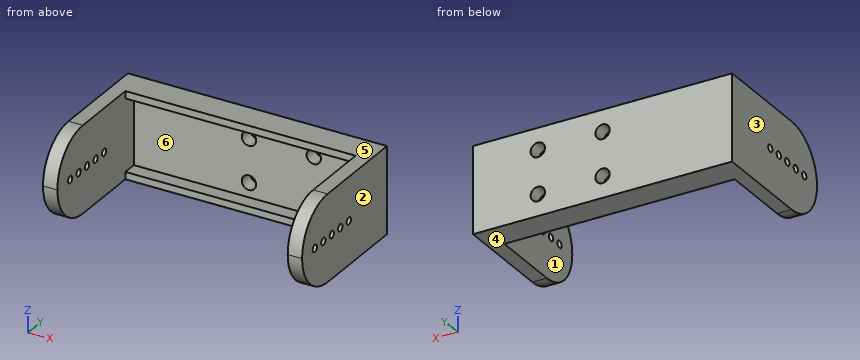
from build123d import *

# Parameters (mm, degrees)
SKETCH1_W           = 36
SKETCH1_H           = 20
BOSS_EXTRUDE1_DEPTH = 12
SKETCH3_W           = 32
SKETCH3_H           = 16
CUT_EXTRUDE1_DEPTH  = 12
SKETCH4_W           = 32
SKETCH4_H           = 12
CUT_EXTRUDE2_DEPTH  = 12
CUT_EXTRUDE3_DEPTH  = 40.242833741
SKETCH5_R           = 1
CUT_EXTRUDE4_DEPTH  = 10
SKETCH6_R           = 0.5
CUT_EXTRUDE5_DEPTH  = 40.242833741
SKETCH7_W           = 32
SKETCH7_H           = 1
BOSS_EXTRUDE2_DEPTH = 2


with BuildPart() as part:
    # Sketch1 → Boss-Extrude1 (new body)
    with BuildSketch(Plane.XY):
        Rectangle(SKETCH1_W, SKETCH1_H)
    extrude(amount=BOSS_EXTRUDE1_DEPTH)

    # Sketch3 → Cut-Extrude1 (cut)
    with BuildSketch(Plane.XY.offset(12)):
        Rectangle(SKETCH3_W, SKETCH3_H)
    extrude(amount=-CUT_EXTRUDE1_DEPTH, mode=Mode.SUBTRACT)

    # Sketch4 → Cut-Extrude2 (cut)
    with BuildSketch(Plane(origin=(0, -8, 0), x_dir=(1, 0, 0), z_dir=(0, 1, 0))):
        with Locations((0, -6)):
            Rectangle(SKETCH4_W, SKETCH4_H)
    extrude(amount=-CUT_EXTRUDE2_DEPTH, mode=Mode.SUBTRACT)

    # Sketch2 → Cut-Extrude3 (cut, through all)
    with BuildSketch(Plane(origin=(18, 0, 0), x_dir=(0, 0, -1), z_dir=(1, 0, 0))):
        with BuildLine():
            Line((-12, -10), (-6, -10))
            ThreePointArc((-6, -10), (-10.242640687, -8.242640687), (-12, -4))
            Line((-12, -4), (-12, -10))
        make_face()
        with BuildLine():
            Line((-6, -10), (0, -10))
            Line((0, -10), (0, -4))
            ThreePointArc((0, -4), (-1.757359313, -8.242640687), (-6, -10))
        make_face()
    extrude(amount=-CUT_EXTRUDE3_DEPTH, mode=Mode.SUBTRACT)

    # Sketch5 → Cut-Extrude4 (cut)
    with BuildSketch(Plane(origin=(0, 10, 0), x_dir=(1, 0, 0), z_dir=(0, 1, 0))):
        with Locations(Location((9, -3, 0), (0, 0, 270))):
            Circle(SKETCH5_R)
        with Locations(Location((9, -9, 0), (0, 0, 180))):
            Circle(SKETCH5_R)
        with Locations(Location((0, -9, 0), (0, 0, 180))):
            Circle(SKETCH5_R)
        with Locations(Location((0, -3, 0), (0, 0, 270))):
            Circle(SKETCH5_R)
    extrude(amount=-CUT_EXTRUDE4_DEPTH, mode=Mode.SUBTRACT)

    # Sketch6 → Cut-Extrude5 (cut, through all)
    with BuildSketch(Plane(origin=(18, 0, 0), x_dir=(0, 0, -1), z_dir=(1, 0, 0))):
        with Locations((-6, -7)):
            Circle(SKETCH6_R)
        with Locations((-6, -5)):
            Circle(SKETCH6_R)
        with Locations((-6, -3)):
            Circle(SKETCH6_R)
        with Locations((-6, -1)):
            Circle(SKETCH6_R)
        with Locations((-6, 1)):
            Circle(SKETCH6_R)
    extrude(amount=-CUT_EXTRUDE5_DEPTH, mode=Mode.SUBTRACT)

    # Sketch7 → Boss-Extrude2 (add)
    with BuildSketch(Plane.XZ.offset(-8)):
        with Locations((0, 11.5)):
            Rectangle(SKETCH7_W, SKETCH7_H)
        with Locations((0, 0.5)):
            Rectangle(SKETCH7_W, SKETCH7_H)
    extrude(amount=BOSS_EXTRUDE2_DEPTH)


solid = part.part
For this review, take the finished solid that the model builds, in its own axes (mm). Face numbers are marked on the shaded views. A direction names the side the tool comes from. Round coordinates to 2 decimals unless told otherwise and drop trailing zeros. Order: outer loops, then holes, each group sorted by start corner. A loop starts at its lowest first (then second) coordinate and runs counter-clockwise, first axis right, second up. Notation, with made-up numbers: (79.5, 22.5) -> (88.5, 22.5) arc R13 ccw to (88.5, 31.5) -> close; hole circle Ø1 at (56, 37). An arc over 180 degrees is marked (long way). Put each result on its own line as item: value.
Q1. Add section C-C on y = -8. Write out the cut boundary in (x, z), plus the area to 3 significant figures.
Check result:
outline: (-18, 1.53) -> (-16, 1.53) -> (-16, 10.47) -> (-18, 10.47) -> close; (16, 1.53) -> (18, 1.53) -> (18, 10.47) -> (16, 10.47) -> close
area: 35.8 mm2
Q2. For probe 1 along X at (y, z) = (8.9, 3); probe 2 along Y at (x, z) = (-17.1, 6); probe 3 along X at (y, z) = (6.5, 6.25), list the stretches that pass through material, from the lowest coordinate up. Write a range as [from, to].
Check result:
probe 1: [-18, -1], [1, 8], [10, 18]
probe 2: [-10, -7.5], [-6.5, -5.5], [-4.5, -3.5], [-2.5, -1.5], [-0.5, 0.5], [1.5, 10]
probe 3: [-18, -16], [16, 18]
Q3. Add section A-A on y = -1. Write out the cut boundary in (x, z).
Check result:
outline: (-18, 0) -> (-16, 0) -> (-16, 5.5) -> (-18, 5.5) -> close; (-18, 6.5) -> (-16, 6.5) -> (-16, 12) -> (-18, 12) -> close; (16, 0) -> (18, 0) -> (18, 5.5) -> (16, 5.5) -> close; (16, 6.5) -> (18, 6.5) -> (18, 12) -> (16, 12) -> close
Q4. Insertion check: pin 1 Ø0.5 at (x, z) = (-4, 0.5) entering from -Y; pin 2 Ø1.6 at (x, z) = (9, 3) entering from -Y; pin 3 Ø3 at (x, z) = (-9, 6.5) entering from -Y. Each pin has a flat end and moves straight along its axis. Give the tip position at first contact, or say it passes through.
Check result:
pin 1: y = 6
pin 2: through
pin 3: y = 8
Q5. Add section D-D on z = 4.5. Write out the cut boundary in (x, y).
Check result:
outline: (-18, -9.81) -> (-16, -9.81) -> (-16, 8) -> (16, 8) -> (16, -9.81) -> (18, -9.81) -> (18, 10) -> (-18, 10) -> close
Q6. Add section B-B on x = 9. Write out the cut boundary in (y, z).
Check result:
outline: (6, 0) -> (10, 0) -> (10, 2) -> (8, 2) -> (8, 1) -> (6, 1) -> close; (6, 11) -> (8, 11) -> (8, 10) -> (10, 10) -> (10, 12) -> (6, 12) -> close; (8, 4) -> (10, 4) -> (10, 8) -> (8, 8) -> close
Q7. Mouldability with a two-part tool opening along X and no side actions: class the marked faces 1, 2, 3 and 4 as pulls with the +X half, pulls with the -X half, needs draft (parallel to the pull), parting line crosses it, or undercut.
Check result:
face 1: undercut
face 2: pulls with the +X half
face 3: pulls with the -X half
face 4: needs draft
Q8. Machinability: for the marked faces 5 and 6, which of the approach directions +Z, -Z, +X, -X, +Y, -Y give a long, thin tool a straight path to every point of the face, cutting with its end or side? Answer none if there is none.
Check result:
face 5: +Z, +X, -X, +Y, -Y
face 6: -Y
